Geometry: see drawing. Coordinates: mm, zero at the bounding-box minimum. Give positions to 0.01 mm unless a question says otherwise; leave off trailing zeros. Loops run counter-clockwise (first coordinate to the right, second up) from the corner with the lowest first, then second, coordinate; pieces in that order, holes last. Notation, with made-up numbers: M 30,20 L 37,20 A16 ccw 37,46 Z; hole C 6,79 d4. An arc over 180 degrees is marked long. Use CSV: the item, a comma, the result in double quotes. Start each with the question number.
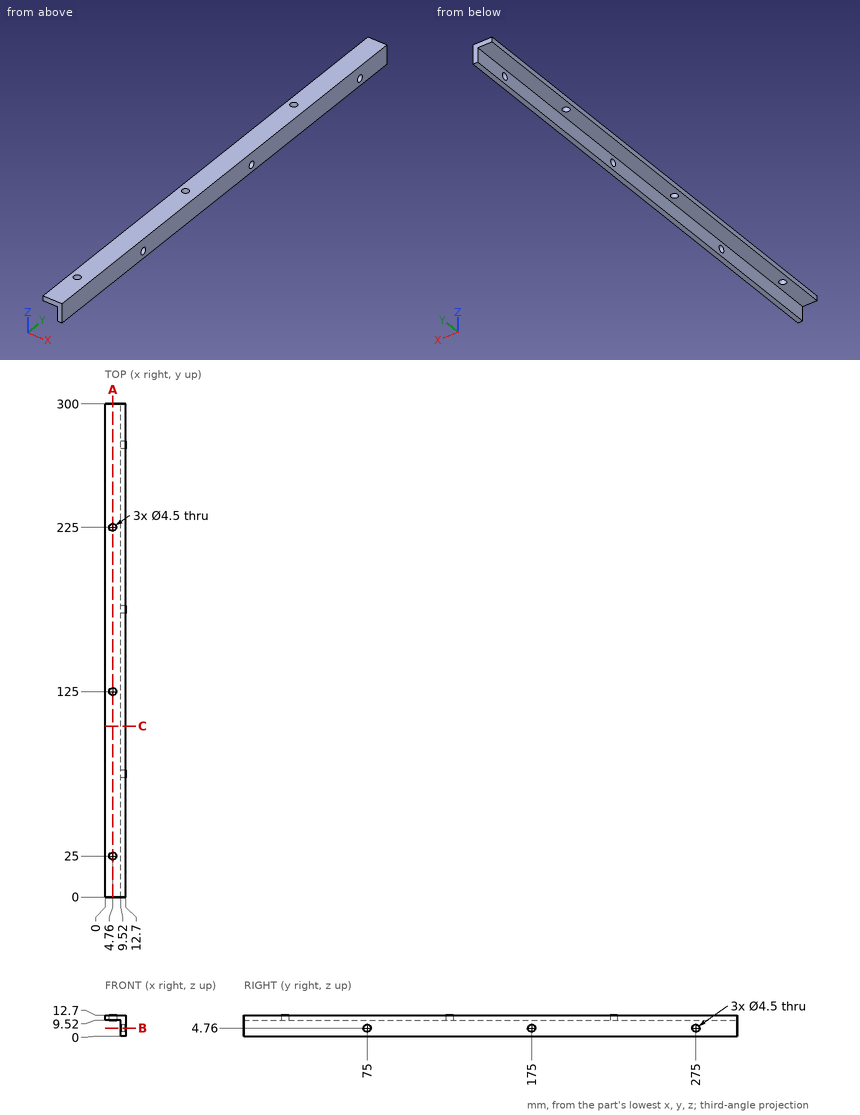
Item 1: Material intervals for line 1 (Y direction, x = 4.76, z = 10.45); line 2 (Y direction, x = 11.45, z = 4.76); line 3 (Z direction, x = 10.9, y = 175), sorted ascending.
Item 2: First-contact query: pin 1 Ø2 at (x, z) = (4, 9) entering from +Y; pin 2 Ø5 at (x, y) = (5, 221) entering from -Z; pin 3 Ø5 at (y, z) = (175, 4.76) entering from -X. Flat tips, straight axial feed; report the tip coordinate or a pass-through.
Item 3: Section C-C (y = 104). Output: boundary loops of the cut face in (x, z).
Item 4: Section A-A (x = 4.76). Output: boundary loops of the cut face in (y, z).
Item 5: Section B-B (z = 4.76). Output: boundary loops of the cut face in (x, y).
Recorded:
1,line 1,"0 to 22.75, 27.25 to 122.75, 127.25 to 222.75, 227.25 to 300"
1,line 2,"0 to 72.75, 77.25 to 172.75, 177.25 to 272.75, 277.25 to 300"
1,line 3,"0 to 2.51, 7.01 to 12.7"
2,pin 1,"y = 300"
2,pin 2,"z = 9.52"
2,pin 3,"x = 9.52"
3,outline,"M 0,9.52 L 9.52,9.52 L 9.52,0 L 12.7,0 L 12.7,12.7 L 0,12.7 Z"
4,outline,"M 0,9.52 L 22.75,9.52 L 22.75,12.7 L 0,12.7 Z; M 27.25,9.52 L 122.75,9.52 L 122.75,12.7 L 27.25,12.7 Z; M 127.25,9.52 L 222.75,9.52 L 222.75,12.7 L 127.25,12.7 Z; M 227.25,9.52 L 300,9.52 L 300,12.7 L 227.25,12.7 Z"
5,outline,"M 9.52,0 L 12.7,0 L 12.7,72.75 L 9.52,72.75 Z; M 9.52,77.25 L 12.7,77.25 L 12.7,172.75 L 9.52,172.75 Z; M 9.52,177.25 L 12.7,177.25 L 12.7,272.75 L 9.52,272.75 Z; M 9.52,277.25 L 12.7,277.25 L 12.7,300 L 9.52,300 Z"
